Geometry: final body of the model. Coordinates: model frame, mm. Coordinates: 2 decimals unless noted, no trailing zeros. Loops run counter-clockwise (first coordinate to the right, second up) from the corner with the lowest first, then second, coordinate; pieces in that order, holes last. Notation, with made-up numbers: (72, -16) -> (97, -16) arc R17 ccw to (97, -8) -> close; hole circle Ø1 at (-38, -16). An arc over 180 degrees is marked (long way). One line per item, written item: value. Start each with the question number.
from build123d import *

# Parameters (mm, degrees)
ESQUISSE1_W             = 165
ESQUISSE1_H             = 15
BOSS_EXTRU_1_DEPTH      = 6
ESQUISSE4_W             = 180.64112288
ESQUISSE4_H             = 30
ENL_V_MAT_EXTRU_1_DEPTH = 12
ESQUISSE3_R             = 1.55
ENL_V_MAT_EXTRU_2_DEPTH = 12
ENL_V_MAT_EXTRU_3_DEPTH = 2


with BuildPart() as part:
    # Esquisse1 → Boss.-Extru.1 (new body)
    with BuildSketch(Plane(origin=(0, 0, 0), x_dir=(1, 0, 0), z_dir=(0, 1, 0))):
        Rectangle(ESQUISSE1_W, ESQUISSE1_H)
    extrude(amount=BOSS_EXTRU_1_DEPTH)

    # Esquisse4 → Enlèv. mat.-Extru.1 (cut)
    with BuildSketch(Plane(origin=(0, 6, 0), x_dir=(1, 0, 0), z_dir=(0, 1, 0))):
        Rectangle(ESQUISSE4_W, ESQUISSE4_H)
        with BuildLine():
            Line((-67.159158072, 7.5), (-64.738516234, 5.079358161))
            Line((-64.738516234, 5.079358161), (64.738516234, 5.079358161))
            Line((64.738516234, 5.079358161), (67.159158072, 7.5))
            Line((67.159158072, 7.5), (75, 7.5))
            add(Edge.make_bspline(
                [(75, 7.5), (79.08518124, 7.773957054), (85.914818759, -1e-09), (79.085181242, -7.773957053), (75, -7.5)],
                knots=[0, 0, 0, 0, 0.5, 1, 1, 1, 1], degree=3))
            Line((75, -7.5), (67.159158072, -7.5))
            Line((67.159158072, -7.5), (64.738516234, -5.079358161))
            Line((64.738516234, -5.079358161), (-64.738516234, -5.079358161))
            Line((-64.738516234, -5.079358161), (-67.159158072, -7.5))
            Line((-67.159158072, -7.5), (-75, -7.5))
            add(Edge.make_bspline(
                [(-75, 7.5), (-79.08518124, 7.773957054), (-85.914818759, -1e-09), (-79.085181242, -7.773957053), (-75, -7.5)],
                knots=[0, 0, 0, 0, 0.5, 1, 1, 1, 1], degree=3))
            Line((-75, 7.5), (-67.159158072, 7.5))
        make_face(mode=Mode.SUBTRACT)
    extrude(amount=-ENL_V_MAT_EXTRU_1_DEPTH, mode=Mode.SUBTRACT)

    # Esquisse3 → Enlèv. mat.-Extru.2 (cut)
    with BuildSketch(Plane.XZ):
        with Locations(Location((-75, 0, 0), (0, 0, 270))):
            Circle(ESQUISSE3_R)
        with Locations(Location((75, 0, 0), (0, 0, 270))):
            Circle(ESQUISSE3_R)
    extrude(amount=-ENL_V_MAT_EXTRU_2_DEPTH, mode=Mode.SUBTRACT)

    # Esquisse5 → Enlèv. mat.-Extru.3 (cut)
    with BuildSketch(Plane(origin=(0, 6, 0), x_dir=(1, 0, 0), z_dir=(0, 1, 0))):
        Polygon((-65.624952607, 0), (-66.717415088, 3.351936497), (66.717415088, 3.351936497), (65.624952607, 0), (66.717415088, -3.351936497), (-66.717415088, -3.351936497), align=None)
    extrude(amount=-ENL_V_MAT_EXTRU_3_DEPTH, mode=Mode.SUBTRACT)


solid = part.part
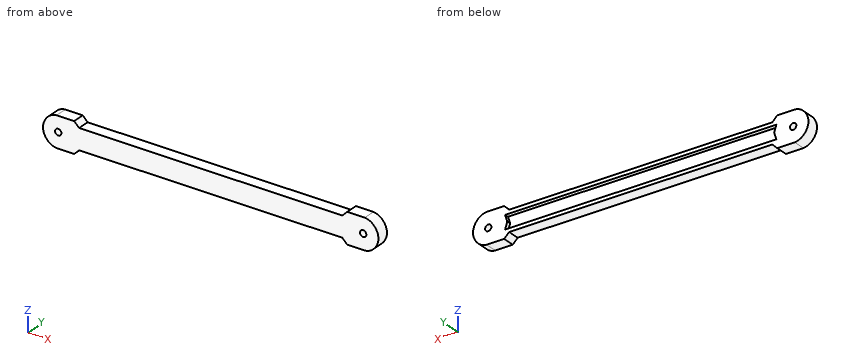
1. Line query: L1, parallel to X at y = 3.15, z = 0; L2, parallel to X at y = 4.3, z = 0; L3, parallel to Z at x = 75, y = 4.6. Output: solid intervals per line, ascending. Write a range as [from, to].
2. Section A-A on x = -25. Return the cut outline in (y, z).
3. Section B-B on y = 1.75. Count the separate pieces of the cut face and the enclosed holes in it, plus the area to 3 significant figures.
4. Pin query (flat end, axial travel): pin 1 Ø3 at (y, z) = (3.5, -6) entering from +X; pin 2 Ø1 at (x, y) = (-32.5, 5) entering from -Z; pin 3 Ø2 at (y, z) = (4, -4) entering from +X; pin 4 Ø3 at (x, z) = (-75, 0) entering from +Y. Return the tip coordinate at first contact, or that it passes through.
Checks:
1. L1: [-82.5, -76.55], [-73.45, 73.45], [76.55, 82.5]
1. L2: [-82.5, -76.55], [-73.45, -65.62], [65.62, 73.45], [76.55, 82.5]
1. L3: [-7.5, -1.55], [1.55, 7.5]
2. outline: (0, -5.08) -> (6, -5.08) -> (6, -3.35) -> (4, -3.35) -> (4, 3.35) -> (6, 3.35) -> (6, 5.08) -> (0, 5.08) -> close
3. separate pieces: 1
3. enclosed holes: 2
3. area: 1,770 mm²
4. pin 1: x = 80.96
4. pin 2: z = -5.08
4. pin 3: x = 81.84
4. pin 4: through
